from build123d import *

# Parameters (mm, degrees)
F2_R          = 11.43
F2_R_2        = 8.89
F0_W          = 177.8
F0_H          = 5.7147379888
F4_DEPTH      = 25.4
F4_DEPTH_BACK = 25.4
F5_DEPTH      = 25.4
F7_R          = 4.445
F8_DEPTH      = 38.1


with BuildPart() as f3:
    # F3: sweep along a path in F0
    with BuildLine(Plane.XY) as f3_path:
        ThreePointArc((140.97, 0), (-140.9612054829, 1.5746265624), (140.9348230289, -3.1490566563))
        ThreePointArc((140.9348230289, -3.1490566563), (140.9612054829, -1.5746265624), (140.97, 0))
    # F2 (on line) → F3 (sweep)
    with BuildSketch(Plane(origin=(0, 0, 0), x_dir=(-1, 0, 0), z_dir=(0, 1, 0))):
        with Locations((-140.97, 0)):
            Circle(F2_R)
        with Locations((-140.97, 0)):
            Circle(F2_R_2, mode=Mode.SUBTRACT)
    sweep(path=f3_path.line)

    # F0 (on Top) → F4 (cut, two sides)
    with BuildSketch(Plane.XY) as f4_sk:
        with BuildLine():
            ThreePointArc((-140.6813228933, -9.017), (-4.5108098905, 140.8978122404), (140.97, 0))
            ThreePointArc((140.97, 0), (140.9612054829, -1.5746265624), (140.9348230289, -3.1490566563))
            ThreePointArc((140.9348230289, -3.1490566563), (15.7764325547, -140.0844212461), (-136.7041001982, -34.417))
            Line((-136.7041001982, -34.417), (-181.8818151951, -34.417))
            Line((-181.8818151951, -34.417), (-181.8818151951, -162.2846722603))
            Line((-181.8818151951, -162.2846722603), (186.068713665, -162.2846722603))
            Line((186.068713665, -162.2846722603), (186.068713665, 166.5027737617))
            Line((186.068713665, 166.5027737617), (-181.8818151951, 166.5027737617))
            Line((-181.8818151951, 166.5027737617), (-181.8818151951, -9.017))
            Line((-181.8818151951, -9.017), (-140.6813228933, -9.017))
        make_face()
        with BuildLine():
            ThreePointArc((-127.517044002, -34.417), (17.359078723, -130.9342918639), (132.08, 0))
            Line((132.08, 0), (94.4372, 0))
            Line((94.4372, 0), (94.4372, -16.0022620112))
            Line((94.4372, -16.0022620112), (94.4372, -21.717))
            Line((94.4372, -21.717), (-83.3628, -21.717))
            Line((-83.3628, -21.717), (-83.3628, -34.417))
            Line((-83.3628, -34.417), (-127.517044002, -34.417))
        make_face()
        with BuildLine():
            Line((94.4372, 0), (132.08, 0))
            ThreePointArc((132.08, 0), (-4.5111319594, 132.0029396962), (-131.7718487045, -9.017))
            Line((-131.7718487045, -9.017), (-83.3628, -9.017))
            Line((-83.3628, -9.017), (-83.3628, -16.0022620112))
            Line((-83.3628, -16.0022620112), (94.4372, -16.0022620112))
            Line((94.4372, -16.0022620112), (94.4372, 0))
        make_face()
        with Locations((5.5372, -18.8596310056)):
            Rectangle(F0_W, F0_H)
        with BuildLine():
            Line((140.97, 0), (132.08, 0))
            ThreePointArc((132.08, 0), (17.359078723, -130.9342918639), (-127.517044002, -34.417))
            Line((-127.517044002, -34.417), (-136.7041001982, -34.417))
            ThreePointArc((-136.7041001982, -34.417), (15.7764325547, -140.0844212461), (140.9348230289, -3.1490566563))
            ThreePointArc((140.9348230289, -3.1490566563), (140.9612054829, -1.5746265624), (140.97, 0))
        make_face()
        with BuildLine():
            ThreePointArc((-131.7718487045, -9.017), (-4.5111319594, 132.0029396962), (132.08, 0))
            Line((132.08, 0), (140.97, 0))
            ThreePointArc((140.97, 0), (-4.5108098905, 140.8978122404), (-140.6813228933, -9.017))
            Line((-140.6813228933, -9.017), (-131.7718487045, -9.017))
        make_face()
    extrude(amount=F4_DEPTH, mode=Mode.SUBTRACT)
    extrude(f4_sk.sketch, amount=-F4_DEPTH_BACK, mode=Mode.SUBTRACT)

    # F0 (on Top) → F5 (cut)
    with BuildSketch(Plane.XY):
        with BuildLine():
            ThreePointArc((-139.2871595338, -21.717), (-140.1281923388, -15.3828024712), (-140.6813228933, -9.017))
            Line((-140.6813228933, -9.017), (-181.8818151951, -9.017))
            Line((-181.8818151951, -9.017), (-198.6888721585, -9.017))
            Line((-198.6888721585, -9.017), (-198.6888721585, -34.417))
            Line((-198.6888721585, -34.417), (-181.8818151951, -34.417))
            Line((-181.8818151951, -34.417), (-136.7041001982, -34.417))
            ThreePointArc((-136.7041001982, -34.417), (-138.1416532481, -28.0966997685), (-139.2871595338, -21.717))
        make_face()
        with BuildLine():
            Line((-83.3628, -9.017), (-131.7718487045, -9.017))
            ThreePointArc((-131.7718487045, -9.017), (-131.1808944972, -15.385035551), (-130.282379127, -21.717))
            Line((-130.282379127, -21.717), (-83.3628, -21.717))
            Line((-83.3628, -21.717), (-83.3628, -16.0022620112))
            Line((-83.3628, -16.0022620112), (-83.3628, -9.017))
        make_face()
        with BuildLine():
            ThreePointArc((-130.282379127, -21.717), (-129.056027141, -28.1010366106), (-127.517044002, -34.417))
            Line((-127.517044002, -34.417), (-83.3628, -34.417))
            Line((-83.3628, -34.417), (-83.3628, -21.717))
            Line((-83.3628, -21.717), (-130.282379127, -21.717))
        make_face()
        with BuildLine():
            Line((-136.7041001982, -34.417), (-127.517044002, -34.417))
            ThreePointArc((-127.517044002, -34.417), (-129.056027141, -28.1010366106), (-130.282379127, -21.717))
            Line((-130.282379127, -21.717), (-139.2871595338, -21.717))
            ThreePointArc((-139.2871595338, -21.717), (-138.1416532481, -28.0966997685), (-136.7041001982, -34.417))
        make_face()
        with BuildLine():
            ThreePointArc((-130.282379127, -21.717), (-131.1808944972, -15.385035551), (-131.7718487045, -9.017))
            Line((-131.7718487045, -9.017), (-140.6813228933, -9.017))
            ThreePointArc((-140.6813228933, -9.017), (-140.1281923388, -15.3828024712), (-139.2871595338, -21.717))
            Line((-139.2871595338, -21.717), (-130.282379127, -21.717))
        make_face()
    extrude(amount=-F5_DEPTH, mode=Mode.SUBTRACT)

    # F7 (on line) → F8 (join)
    with BuildSketch(Plane(origin=(-139.2871595338, 0, 0), x_dir=(0, -1, 0), z_dir=(-1, 0, 0))):
        with Locations((21.717, 0)):
            Circle(F7_R)
    extrude(amount=-F8_DEPTH)


solid = f3.part
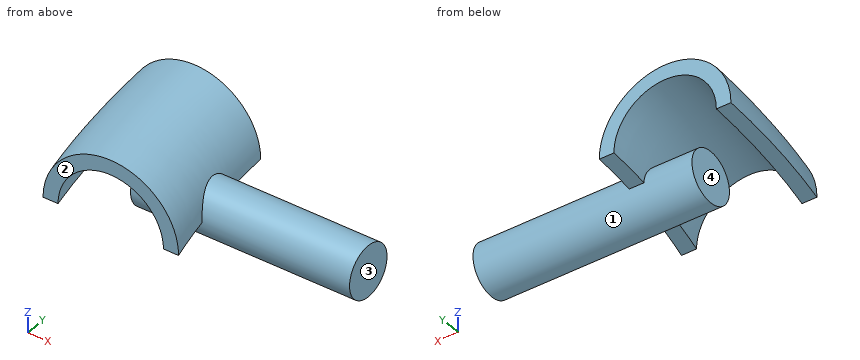
Geometry: final body of the model. Coordinates: model frame, mm. Face numbers are marked on the shaded views. Give positions to 0.01 mm unless a question says otherwise; leave off trailing zeros. Order: outer loops, then holes, each group sorted by start corner. A loop starts at its lowest first (then second) coordinate and runs counter-clockwise, first axis right, second up. Notation, with made-up numbers: (38, 78.25) -> (68, 78.25) arc R17 cw to (68, 84.25) -> close; hole circle Ø6 at (4.25, 89.25). An arc over 180 degrees is marked (long way). Answer as a JSON object with one key per item and string values.
Q1. Material intervals for probe 1 along X at (y, z) = (-28.5, 2); probe 2 along X at (y, z) = (-32.25, 6.5); probe 3 along Y at (x, z) = (-134.5, 0), sorted ascending.
Entries:
{"probe 1": "x = -149.53 to -146.89, -129.2 to -126.55", "probe 2": "x = -146.87 to -143.45, -130.99 to -127.55", "probe 3": "y = -26.16 to -17.27"}
Q2. Section A-A (z = 7). Output: boundary loops of the cut face in (x, y), plus the area to 3 significant figures.
Entries:
{"outline": "(-149.73, -9.02) arc R150.01 ccw to (-146, -34.42) -> (-142.35, -34.42) arc R146.45 cw to (-146.17, -9.02) -> close; (-135.19, -9.02) arc R135.49 ccw to (-131.05, -34.42) -> (-127.37, -34.42) arc R131.93 cw to (-131.63, -9.02) -> close", "area": "183 mm^2"}
Q3. Section B-B (x = -108.5). Output: boundary loops of the cut face in (y, z) (3 decimals).
Entries:
{"outline": "circle Ø8.89 at (-21.717, 0)"}
Q4. First-contact query: pin 1 (1 mm diameter, centred on y = -26, z = -1.5, fed in from +X); pin 2 (7 mm diameter, centred on y = -21, z = -1, fed in from -X) (3 decimals); pin 3 (4 mm diameter, centred on x = -109, y = -18, fed in from +Z); pin 4 (1.7 mm diameter, centred on x = -130.5, y = -12, fed in from -Z). Flat tips, straight axial feed; report the tip coordinate or a pass-through.
Entries:
{"pin 1": "stops at x = -101.19", "pin 2": "stops at x = -151.375", "pin 3": "stops at z = 4.1", "pin 4": "stops at z = 0"}
Q5. Draft query along X for the marked faces 1, 2, 3 and 4. Return one class per face: released by +X, released by -X, zero draft, split by the parting line, or undercut.
Entries:
{"face 1": "undercut", "face 2": "zero draft", "face 3": "released by +X", "face 4": "undercut"}
